Check sheet for the modelled part. Datum: model origin and axes. Units: mm. Round coordinates to 2 decimals unless told otherwise and drop trailing zeros. Write each loop counter-clockwise with the first axis right and the second up, starting at its lowest first coordinate (ties: lowest second). Pieces come first, ordered by that corner, then holes. Notation, with made-up numbers: (-34.75, 22.25) -> (21.25, 22.25) arc R18 ccw to (21.25, 29.25) -> close; hole circle Ø9 at (-36.5, 20.25). An arc over 180 degrees is marked (long way). One line per item, written item: value. Start each with the question number.
Autodesk Inventor part; units mm, degrees
ref_plane "工作平面1" through (0, 40, 20) normal (-0.2294, 0.6882, 0.6882) x (0, -0.7071, 0.7071)
ref_plane "工作平面3" through (0, 40, 0) normal (0.2294, 0.6882, -0.6882) x (0.9487, 0, 0.3162)
ref_plane "YZ Plane" through (0, 0, 0) normal (1, 0, 0) x (0, 1, 0)
sketch "草圖1" plane through (0, 0, 0) normal (0, 0, 1) x (1, 0, 0)
  line L0 (-12, 0) -> (72, 0)
  line L1 (0, -8) -> (0, 48)
  line L2 (0, 0) -> (60, 0)
  line L3 (60, 0) -> (60, 40)
  line L4 (60, 40) -> (0, 40)
  line L5 (0, 40) -> (0, 0)
  dimension "d0" = 60
  dimension "d1" = 40
extrude "擠出1" add sketch "草圖1" along normal blind 40
ref_plane "工作平面1" through (0, 40, 20) normal (-0.2294, 0.6882, 0.6882) x (0, -0.7071, 0.7071)
sketch "草圖2" plane through (0, 40, 20) normal (-0.2294, 0.6882, 0.6882) x (0, -0.7071, 0.7071)
  line L0 (42.4264, 55.1553) -> (14.1421, 61.6441)
  line L1 (14.1421, 3.2444) -> (42.4264, -3.2444)
  line L2 (-14.1421, -3.2444) -> (14.1421, 3.2444)
  line L3 (-24.1266, -29.4243) -> (37.1709, -29.4243)
  line L4 (37.1709, -29.4243) -> (37.1709, 87.3992)
  line L5 (37.1709, 87.3992) -> (-24.1266, 87.3992)
  line L6 (-24.1266, 87.3992) -> (-24.1266, -29.4243)
  point P0 (14.1421, -9.7333)
extrude "擠出2" cut sketch "草圖2" along normal blind 40
ref_plane "工作平面3" through (0, 40, 0) normal (0.2294, 0.6882, -0.6882) x (0.9487, 0, 0.3162)
sketch "草圖4" plane through (0, 40, 0) normal (0.2294, 0.6882, -0.6882) x (0.9487, 0, 0.3162)
  line L0 (-18.5971, -44.6398) -> (132.4913, -44.6398)
  line L1 (132.4913, -44.6398) -> (132.4913, 100.0809)
  line L2 (132.4913, 100.0809) -> (-18.5971, 100.0809)
  line L3 (-18.5971, 100.0809) -> (-18.5971, -44.6398)
  point P0 (0, 29.0191)
extrude "擠出4" cut sketch "草圖4" along normal blind 40
1. Cross-section at C-C (y = 29). Record the cut outline in (x, z), plus the area to 3 significant figures.
2. Cross-section at D-D (z = 25). Record the cut outline in (x, y), plus the area to 3 significant figures.
3. Release check for a two-part mould opening along Z. For faces 1 (the face through (37.955, 34.304, 6.959)), 2 (the face through (60, 20, 20)), 3 (the face through (30, 16, 40)) record: +Z half, -Z half, draft (parallel to the pull), parting line (faces both ways), or undercut.
4. Depth check by flat-ended pin: pin 1 Ø1.5 at (x, z) = (34.5, 35.5) entering from +Y. Enter the tip coordinate at first touch or a pass-through.
5. Cross-section at A-A (z = 3.5). Record the cut outline in (x, y).
6. Cross-section at B-B (x = 46). Record the cut outline in (y, z).
7. Material ranges on probe 1 along Y at (x, z) = (33.5, 35); probe 2 along Z at (x, y) = (53.5, 30.5); probe 3 along Z at (x, y) = (23.5, 34), recorded low to high.
Working result:
1. outline: (0, 0) -> (32.99, 0) -> (60, 9) -> (60, 40) -> (27.01, 40) -> (0, 31) -> close
1. area: 2,160 mm^2
2. outline: (0, 0) -> (60, 0) -> (60, 40) -> (15.01, 40) -> (0, 35) -> close
2. area: 2,360 mm^2
3. face 1: -Z half
3. face 2: draft
3. face 3: +Z half
4. pin 1: stops at y = 36.79
5. outline: (0, 0) -> (60, 0) -> (60, 23.5) -> (10.49, 40) -> (0, 40) -> close
6. outline: (0, 0) -> (24.66, 0) -> (40, 15.34) -> (40, 35.33) -> (35.33, 40) -> (0, 40) -> close
7. probe 1: y = 0 to 36.16
7. probe 2: z = 8.34 to 40
7. probe 3: z = 1.84 to 33.83
